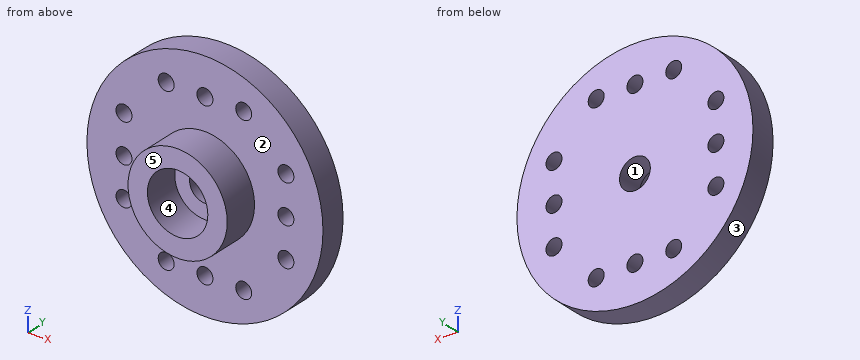
```python
from build123d import *

# Parameters (mm, degrees)
SKETCH1_R           = 10.35
BOSS_EXTRUDE1_DEPTH = 2.28
SKETCH2_R           = 4.35
BOSS_EXTRUDE2_DEPTH = 3.1
SKETCH3_R           = 1.35
CUT_EXTRUDE1_DEPTH  = 6.38
SKETCH4_R           = 2.65
CUT_EXTRUDE2_DEPTH  = 3.1
SKETCH5_R           = 0.7
CUT_EXTRUDE3_DEPTH  = 3.1
CIRPATTERN1_COUNT   = 4


with BuildPart() as part:
    # Sketch1 → Boss-Extrude1 (new body)
    with BuildSketch(Plane(origin=(0, 0, 0), x_dir=(1, 0, 0), z_dir=(0, 1, 0))):
        Circle(SKETCH1_R)
    extrude(amount=-BOSS_EXTRUDE1_DEPTH)

    # Sketch2 → Boss-Extrude2 (add)
    with BuildSketch(Plane.XZ.offset(2.28)):
        Circle(SKETCH2_R)
    extrude(amount=BOSS_EXTRUDE2_DEPTH)

    # Sketch3 → Cut-Extrude1 (cut, through all)
    with BuildSketch(Plane(origin=(0, 0, 0), x_dir=(1, 0, 0), z_dir=(0, 1, 0))):
        Circle(SKETCH3_R)
    extrude(amount=-CUT_EXTRUDE1_DEPTH, mode=Mode.SUBTRACT)

    # Sketch4 → Cut-Extrude2 (cut)
    with BuildSketch(Plane.XZ.offset(5.38)):
        Circle(SKETCH4_R)
    extrude(amount=-CUT_EXTRUDE2_DEPTH, mode=Mode.SUBTRACT)

    # Sketch5 → Cut-Extrude3 (cut)
    with BuildSketch(Plane(origin=(0, 0, 0), x_dir=(1, 0, 0), z_dir=(0, 1, 0))):
        with Locations((7.1, 3.4)):
            Circle(SKETCH5_R)
        with Locations((7.1, 0)):
            Circle(SKETCH5_R)
        with Locations((7.1, -3.4)):
            Circle(SKETCH5_R)
    cut_extrude3 = extrude(amount=-CUT_EXTRUDE3_DEPTH, mode=Mode.SUBTRACT)

    # CirPattern1: Cut-Extrude3 ×4 about axis
    cirpattern1_axis = Axis((0, 0, 0), (0, 1, 0))
    for i in range(1, CIRPATTERN1_COUNT):
        add(cut_extrude3.rotate(cirpattern1_axis, i * 360 / CIRPATTERN1_COUNT), mode=Mode.SUBTRACT)


solid = part.part
```
Geometry: final body of the model. Coordinates: model frame, mm. Face numbers are marked on the shaded views. A direction names the side the tool comes from. Coordinates: 2 decimals unless noted, no trailing zeros. Order: outer loops, then holes, each group sorted by start corner. A loop starts at its lowest first (then second) coordinate and runs counter-clockwise, first axis right, second up. Notation, with made-up numbers: (-35.75, 0.5) -> (-1.75, 0.5) arc R24 ccw to (-1.75, 13.5) -> close; hole circle Ø9 at (-32.5, -22). An arc over 180 degrees is marked (long way). Use CSV: the item, a comma, the result in double quotes.
1) Section C-C on x = 3.4. Output: boundary loops of the cut face in (y, z).
Findings:
outline,"(-5.38, -2.71) -> (-2.28, -2.71) -> (-2.28, -6.4) -> (0, -6.4) -> (0, 6.4) -> (-2.28, 6.4) -> (-2.28, 2.71) -> (-5.38, 2.71) -> close; (-2.28, -9.78) -> (0, -9.78) -> (0, -7.8) -> (-2.28, -7.8) -> close; (-2.28, 7.8) -> (0, 7.8) -> (0, 9.78) -> (-2.28, 9.78) -> close"
2) Section A-A on x = 0. Output: boundary loops of the cut face in (y, z), then the cut area to 3 significant figures.
Findings:
outline,"(-5.38, -4.35) -> (-2.28, -4.35) -> (-2.28, -6.4) -> (0, -6.4) -> (0, -1.35) -> (-2.28, -1.35) -> (-2.28, -2.65) -> (-5.38, -2.65) -> close; (-5.38, 2.65) -> (-2.28, 2.65) -> (-2.28, 1.35) -> (0, 1.35) -> (0, 6.4) -> (-2.28, 6.4) -> (-2.28, 4.35) -> (-5.38, 4.35) -> close; (-2.28, -10.35) -> (0, -10.35) -> (0, -7.8) -> (-2.28, -7.8) -> close; (-2.28, 7.8) -> (0, 7.8) -> (0, 10.35) -> (-2.28, 10.35) -> close"
area,"45.2 mm^2"
3) Mould query, pull axis Z, two halves, no side actions, for the marked faces 3, 4 and 5. Classes: +Z half, -Z half, draft (parallel to the pull), parting line (faces both ways), or undercut.
Findings:
face 3,"parting line"
face 4,"undercut"
face 5,"draft"
4) Line query: line 1 (X direction, y = -0.65, z = 7.1); line 2 (Y direction, x = 5.75, z = -5.5). Output: solid intervals per line, ascending.
Findings:
line 1,"x = -7.53 to -4.1, -2.7 to -0.7, 0.7 to 2.7, 4.1 to 7.53"
line 2,"y = -2.28 to 0"
5) Section D-D on z = 7.5. Output: boundary loops of the cut face in (x, y).
Findings:
outline,"(-7.13, -2.28) -> (-3.97, -2.28) -> (-3.97, 0) -> (-7.13, 0) -> close; (-2.83, -2.28) -> (-0.57, -2.28) -> (-0.57, 0) -> (-2.83, 0) -> close; (0.57, -2.28) -> (2.83, -2.28) -> (2.83, 0) -> (0.57, 0) -> close; (3.97, -2.28) -> (7.13, -2.28) -> (7.13, 0) -> (3.97, 0) -> close"
6) Pin query (flat end, axial travel): pin 1 Ø6 at (x, z) = (0, 0) entering from -Y; pin 2 Ø2 at (x, z) = (-7.1, 3.4) entering from -Y; pin 3 Ø1.3 at (x, z) = (3.4, -7.1) entering from -Y; pin 4 Ø3 at (x, y) = (4, -2.5) entering from +Z. Return the tip coordinate at first contact, or that it passes through.
Findings:
pin 1,"stops at y = -5.38"
pin 2,"stops at y = -2.28"
pin 3,"passes through"
pin 4,"stops at z = 10.04"
7) Access query for the marked faces 1 and 2. Directions: +Z, -Z, +X, -X, +Y, -Y. A direction counts if a zero-diameter tool reaches every point of the face in a straight line with its end or side. Return the directions, or none.
Findings:
face 1,"+Y, -Y"
face 2,"-Y"
8) Section B-B on y = -2. State how many separate pieces and enclosed holes the cut face has, then the cut area to 3 significant figures.
Findings:
separate pieces,"1"
enclosed holes,"13"
area,"312 mm^2"
